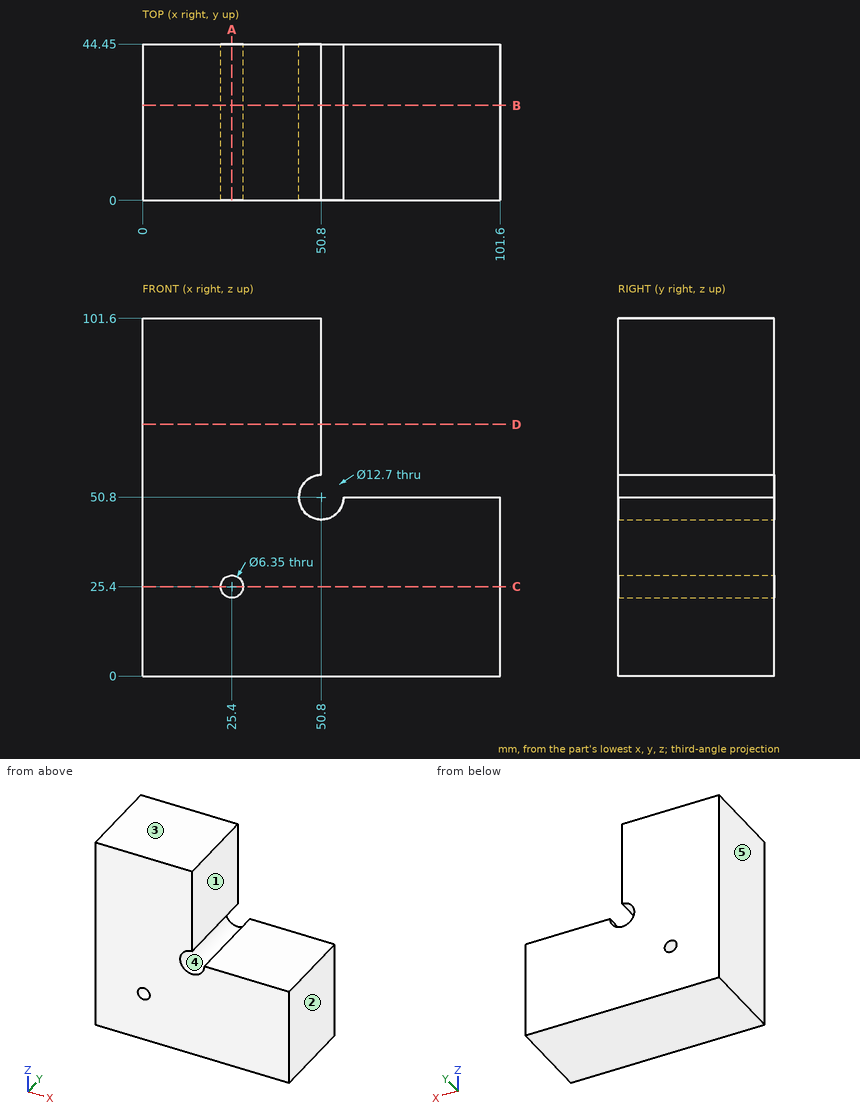
The drawing under review shows one solid part. Ordinate dimensions are in mm from its lowest x, y, z. A direction names the side the tool comes from. Round coordinates to 2 decimals unless told otherwise and drop trailing zeros. Write each loop counter-clockwise with the first axis right and the second up, starting at its lowest first coordinate (ties: lowest second). Pieces come first, ordered by that corner, then holes. Notation, with made-up numbers: (41.5, 14.25) - (55.5, 14.25) arc R30 ccw to (55.5, 44.25) - close; hole circle Ø4 at (2, 88.25). An arc over 180 degrees is marked (long way). Write each question's results on one line, items separated by ' | '.
Item 1: For pin 1 (13.5 mm diameter, centred on x = 70, y = 21, fed in from +Z); pin 2 (1.5 mm diameter, centred on y = 31.5, z = 87.5, fed in from +X), all flat-tipped, find the tip position at first contact; note any pin that passes through.
Calculated:
pin 1: stops at z = 50.8 | pin 2: stops at x = 50.8
Item 2: To check wall thickness, follow line 1 along X through (y, z) = (11, 25); line 2 along Z through (x, y) = (74, 16). State the ranges of each line that lie inside material, in increasing order. Write a range as from..to.
Calculated:
line 1: x = 0..22.25, 28.55..101.6 | line 2: z = 0..50.8
Item 3: Take a section at A-A on x = 25.4. State the section outline as (y, z) points (3 decimals).
Calculated:
outline: (0, 0) - (44.45, 0) - (44.45, 22.225) - (0, 22.225) - close; (0, 28.575) - (44.45, 28.575) - (44.45, 101.6) - (0, 101.6) - close
Item 4: Take a section at B-B on y = 27. State the section outline as (x, z) points (3 decimals), then the cut area to 3 significant figures.
Calculated:
outline: (0, 0) - (101.6, 0) - (101.6, 50.8) - (57.15, 50.8) arc R6.35 cw (long way) to (50.8, 57.15) - (50.8, 101.6) - (0, 101.6) - close; hole circle Ø6.35 at (25.4, 25.4) | area: 7,620 mm^2
Item 5: Draft analysis for pull direction X (two halves, no side actions). For the marked faces 3, 4 and 5, state which applies: pulls with the +X half, pulls with the -X half, needs draft (parallel to the pull), parting line crosses it, or undercut.
Calculated:
face 3: needs draft | face 4: undercut | face 5: pulls with the -X half
Item 6: Take a section at D-D on z = 71.5. State the section outline as (x, y) points, then the cut area to 3 significant figures.
Calculated:
outline: (0, 0) - (50.8, 0) - (50.8, 44.45) - (0, 44.45) - close | area: 2,260 mm^2
Item 7: Take a section at C-C on z = 25.4. State the section outline as (x, y) points (3 decimals), then the cut area to 3 significant figures.
Calculated:
outline: (0, 0) - (22.225, 0) - (22.225, 44.45) - (0, 44.45) - close; (28.575, 0) - (101.6, 0) - (101.6, 44.45) - (28.575, 44.45) - close | area: 4,230 mm^2
Item 8: For the marked faces 1 and 2, list the 3-axis set-ups (+Z, -Z, +X, -X, +Y, -Y) from which the entire face can be reached by the end or side of a thin tool; tool diameter is ignored.
Calculated:
face 1: +Z, +X, +Y, -Y | face 2: +Z, -Z, +X, +Y, -Y
